Source: CAD feature listing. Evaluate the final solid. Frame: model axes, mm. A direction names the side the tool comes from. Give positions to 0.01 mm unless a question says otherwise; leave off trailing zeros. Order: outer loops, then holes, each group sorted by start corner. A loop starts at its lowest first (then second) coordinate and runs counter-clockwise, first axis right, second up.
from build123d import *

# Parameters (mm, degrees)
F0_W     = 914.4
F0_H     = 914.4
F1_DEPTH = 25.4
F2_W     = 254
F2_H     = 254
F3_DEPTH = 1524
F5_DEPTH = 584.201
F6_W     = 304.8
F6_H     = 415.925
F7_DEPTH = 19.05


with BuildPart() as f1:
    # F0 (on Top) → F1 (new body)
    with BuildSketch(Plane.XY):
        with Locations((457.2, 457.2)):
            Rectangle(F0_W, F0_H)
    extrude(amount=F1_DEPTH)

    # F2 (on face) → F3 (join)
    with BuildSketch(Plane.XY.offset(25.4)):
        with Locations((457.2, 787.4)):
            Rectangle(F2_W, F2_H)
    extrude(amount=F3_DEPTH)

    # F4 (on face) → F5 (cut, through all)
    with BuildSketch(Plane.YZ.offset(584.2)):
        Polygon((660.4, 1295.4), (914.4, 1549.4), (660.4, 1549.4), align=None)
    extrude(amount=-F5_DEPTH, mode=Mode.SUBTRACT)

    # F6 (on face) → F7 (join)
    with BuildSketch(Plane(origin=(0, -317.5, 317.5), x_dir=(1, 0, 0), z_dir=(0, -0.707107, 0.707107))):
        with Locations((457.2, 1565.521943)):
            Rectangle(F6_W, F6_H)
    extrude(amount=F7_DEPTH)


solid = f1.part
(1) Section C-C, the plane y = 720. Return loops of the section in (x, z), plus the area to 3 significant figures.
(2) Pin query (flat end, axial travel): pin 1 Ø1 at (x, y) = (237, 132) entering from +Z. Return the tip coordinate at first contact, or that it passes through.
(3) Section D-D, the plane z = 666.5. Return loops of the section in (x, y).
(4) Section B-B, the plane z = 1325.5. Return loops of the section in (x, y).
(5) Access query for faces 1 (the flat face through (455, 914.4, 714)), 2 (the flat face through (584.2, 786, 777)), 3 (the flat face through (321, 790, 1425)), 4 (the flat face through (330.2, 786, 777)), 5 (the flat face through (609.6, 781, 1429)). Directions: +Z, -Z, +X, -X, +Y, -Y. A direction counts if a zero-diameter tool reaches every point of the face in a straight line with its end or side. Return the directions, or none.
(6) Section A-A, the plane x = 478.5. Return loops of the section in (y, z).
(7) Draft query along Z for faces 6 (the flat face through (451, 464, 0)), 7 (the flat face through (304.8, 781, 1429)), 8 (the flat face through (455, 660.4, 652)), 9 (the flat face through (455.07, 778.08, 1440.02)). Return one class per face: +Z half, -Z half, draft (parallel to the pull), parting line (faces both ways), or undercut.
(8) Line query: line 1 along X through (y, z) = (853.5, 162); line 2 along Z through (x, y) = (834.5, 434.5); line 3 along Y through (x, z) = (542, 973.5). Output: solid intervals per line, ascending.
Checks:
1. outline: (0, 0) - (914.4, 0) - (914.4, 25.4) - (584.2, 25.4) - (584.2, 1355) - (609.6, 1355) - (609.6, 1381.94) - (304.8, 1381.94) - (304.8, 1355) - (330.2, 1355) - (330.2, 25.4) - (0, 25.4) - close
1. area: 369,000 mm2
2. pin 1: stops at z = 25.4
3. outline: (330.2, 660.4) - (584.2, 660.4) - (584.2, 914.4) - (330.2, 914.4) - close
4. outline: (304.8, 663.56) - (609.6, 663.56) - (609.6, 690.5) - (584.2, 690.5) - (584.2, 914.4) - (330.2, 914.4) - (330.2, 690.5) - (304.8, 690.5) - close
5. face 1: -Z, +X, -X, +Y
5. face 2: +X, +Y
5. face 3: none
5. face 4: -X, +Y
5. face 5: +Z, +X, +Y, -Y
6. outline: (0, 0) - (914.4, 0) - (914.4, 1549.4) - (936.54, 1571.54) - (923.07, 1585.01) - (628.97, 1290.91) - (642.44, 1277.44) - (660.4, 1295.4) - (660.4, 25.4) - (0, 25.4) - close
7. face 6: -Z half
7. face 7: draft
7. face 8: undercut
7. face 9: +Z half
8. line 1: x = 330.2 to 584.2
8. line 2: z = 0 to 25.4
8. line 3: y = 660.4 to 914.4
